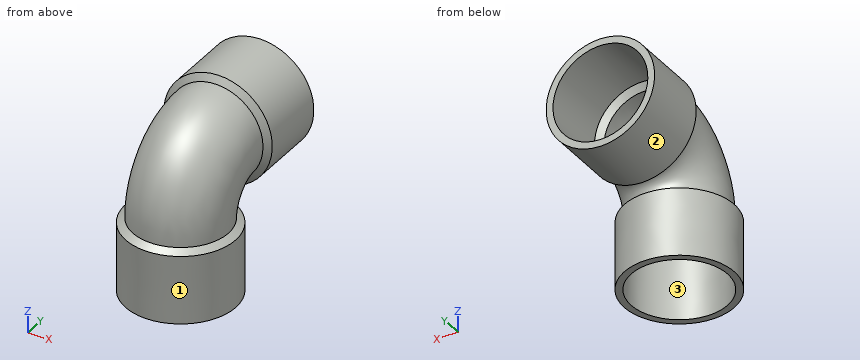
```python
from build123d import *

# Parameters (mm, degrees)
SKETCH1_R      = 21.055
SKETCH1_R_2    = 18.055
REVOLVE1_ANGLE = 90
SKETCH14_W     = 3
SKETCH14_H     = 30
SCALE1_SCALE   = 0.760151086


with BuildPart() as part:
    # Sketch1 → Revolve1 (revolve)
    with BuildSketch(Plane(origin=(0, 0, 0), x_dir=(1, 0, 0), z_dir=(0, 1, 0))):
        Circle(SKETCH1_R)
        Circle(SKETCH1_R_2, mode=Mode.SUBTRACT)
    revolve(axis=Axis((-39.148672595, 0, -25), (1, 0, 0)), revolution_arc=REVOLVE1_ANGLE)

    # Sketch14 → Revolve3 (revolve)
    with BuildSketch(Plane(origin=(0, 0, 0), x_dir=(0, 0, -1), z_dir=(1, 0, 0)), mode=Mode.PRIVATE) as revolve3_sk:
        Polygon((-23.925834548, 2), (-20.925834548, 2), (-17.922072033, 0), (-20.922072033, 0), align=None)
        with Locations((-22.425834548, 17)):
            Rectangle(SKETCH14_W, SKETCH14_H)
    revolve(revolve3_sk.sketch.rotate(Axis((0, 0, 0), (0, 1, 0)), 180), axis=Axis((0, 0, 0), (0, 1, 0)))

    # Sketch20 → Revolve4 (revolve)
    with BuildSketch(Plane(origin=(0, 0, 0), x_dir=(0, 0, -1), z_dir=(1, 0, 0)), mode=Mode.PRIVATE) as revolve4_sk:
        Polygon((27, -49.217355789), (57, -49.26533892), (57, -46.26533892), (27, -46.217355789), align=None)
        Polygon((25, -46.055), (27, -49.217355789), (27, -46.217355789), (25, -43.055), align=None)
    revolve(revolve4_sk.sketch.rotate(Axis((0, -25, -25), (0, 0, -1)), 270), axis=Axis((0, -25, -25), (0, 0, -1)))


with BuildPart() as part_1:
    # Scale1: scaled about (0, -10.246924986, -14.93985455)
    add(part.part.scale(SCALE1_SCALE).moved(Location((0, -2.45771383, -3.583307889))))


solid = part_1.part
```
Work out the finished part from the listing and answer in its coordinate system (mm). Face numbers are marked on the shaded views. Give positions to 0.01 mm unless a question says otherwise; leave off trailing zeros. Loops run counter-clockwise (first coordinate to the right, second up) from the corner with the lowest first, then second, coordinate; pieces in that order, holes last. Notation, with made-up numbers: (25.25, -14.75) -> (55.25, -14.75) arc R15 ccw to (55.25, -2.75) -> close; hole circle Ø7 at (76, 26). An arc over 180 degrees is marked (long way). Write item = value, one per line. Start each with the question number.
(1) The mould has two halves that part along Y. Classify the marked faces 1, 2 and 3: +Y half, -Y half, draft (parallel to the pull), parting line (faces both ways), or undercut.
(2) Find the intervals of material crossed by probe 1 along Y at (x, z) = (11.5, -17); probe 2 along Z at (x, y) = (0.5, -4); probe 3 along Z at (x, y) = (-10, -3), in increasing order. Write a range as from..to.
(3) Find section B-B on z = -36.5. Give the vertices of the cut face in (x, y), and give its area (3 significant figures).
(4) Given pin 1 Ø1.5 at (x, z) = (3, -5.5) entering from -Y; pin 2 Ø13.5 at (x, z) = (-5, -10.5) entering from -Y; pin 3 Ø4 at (x, z) = (-8, 0.5) entering from +Y, each flat-ended and moving along its own axis, determine where each tip first touches the part or whether it passes through.
(5) Find section A-A on y = 15. Give the vertices of the cut face in (x, z), and give its area (3 significant figures).
From the geometry:
q1.face_1 = parting line
q1.face_2 = draft
q1.face_3 = undercut
q2.probe_1 = -32.07..-28.36, -12.52..-8, -1.28..21.87
q2.probe_2 = -46.91..-23.51, -20.01..-17.53, 10.1..12.38
q2.probe_3 = -16.1..-13, 5.81..8.91
q3.outline = circle Ø36.86 at (0, -21.46); hole circle Ø32.3 at (0, -21.46)
q3.area = 248 mm^2
q4.pin_1 = -33.13
q4.pin_2 = -36.82
q4.pin_3 = -17.95
q5.outline = circle Ø36.37 at (0, -3.58); hole circle Ø31.81 at (0, -3.58)
q5.area = 244 mm^2
